from build123d import *

# Parameters (mm, degrees)
SKETCH1_R                 = 8
SKETCH1_R_2               = 11
BOSS_EXTRUDE1_DEPTH       = 5
BOSS_EXTRUDE2_DEPTH       = 11
BOSS_EXTRUDE3_OUTLINE_R   = 1.6
BOSS_EXTRUDE3_OUTLINE_R_2 = 2.1
BOSS_EXTRUDE3_DEPTH       = 3
SKETCH3_W                 = 15
SKETCH3_H                 = 38.75
CUT_EXTRUDE1_DEPTH        = 3
BOSS_EXTRUDE4_REACH       = 120.779
CUT_EXTRUDE3_START        = 3
CUT_EXTRUDE3_OUTLINE_R    = 1.6
CUT_EXTRUDE3_DEPTH        = 5.935416332


# Read off the part's stored shape, not the designer's step: Boss-Extrude3, Cut-Extrude3
with BuildPart() as part:
    # Sketch1 → Boss-Extrude1 (new body)
    with BuildSketch(Plane.XY):
        Polygon((-24, 15), (0, 15), (0, 0), (93, 0), (93, 102.7), (0, 102.7), (0, 30), (-24, 30), align=None)
        with Locations((15, 10.5)):
            Circle(SKETCH1_R, mode=Mode.SUBTRACT)
        with Locations((70, 72)):
            Circle(SKETCH1_R_2, mode=Mode.SUBTRACT)
    extrude(amount=BOSS_EXTRUDE1_DEPTH)

    # Sketch2 → Boss-Extrude2 (add)
    with BuildSketch(Plane(origin=(-11, 0, 0), x_dir=(0, 0, -1), z_dir=(1, 0, 0))):
        Polygon((-6.40446571, 53.75), (-6.40446571, 33.5), (-6.40446571, 30), (0, 30), (0, 53.75), align=None)
    extrude(amount=BOSS_EXTRUDE2_DEPTH)

    # Boss-Extrude3 outline → Boss-Extrude3 (add)
    with BuildSketch(Plane(origin=(-11, 0, 0), x_dir=(0, 0, -1), z_dir=(1, 0, 0))):
        Polygon((-65.7, 15), (-5, 15), (-5, 30), (-6.40446571, 30), (-6.40446571, 53.75), (-65.7, 53.75), align=None)
        with Locations((-25.458037139, 18.009888358)):
            Circle(BOSS_EXTRUDE3_OUTLINE_R, mode=Mode.SUBTRACT)
        with Locations((-33.128928451, 20.361955525)):
            Circle(BOSS_EXTRUDE3_OUTLINE_R_2, mode=Mode.SUBTRACT)
        with BuildLine():
            ThreePointArc((-36.471534651, 41.421088598), (-34.422063775, 42.316430041), (-32.214396715, 42.674443066))
            add(Edge.make_bspline(
                [(-32.214396715, 42.674443066), (-32.258484047, 42.672889926), (-32.30288803, 42.678244048), (-32.383949881, 42.711721435), (-32.420720422, 42.742067925), (-32.450943892, 42.825768035), (-32.442187299, 42.872669516), (-32.401895098, 42.950423281), (-32.37149194, 42.983188581), (-32.336739051, 43.010347732)],
                knots=[0, 0, 0, 0, 0.25, 0.25, 0.5, 0.5, 0.75, 0.75, 1, 1, 1, 1], degree=3))
            ThreePointArc((-32.336739051, 43.010347732), (-12.84214513, 33.068927831), (-32.99665635, 24.544451349))
            add(Edge.make_bspline(
                [(-32.99665635, 24.544451349), (-33.029388791, 24.574028225), (-33.057393425, 24.608892702), (-33.092046693, 24.689435058), (-33.097377316, 24.736767464), (-33.061272852, 24.818024197), (-33.022299349, 24.845743133), (-32.93918463, 24.87327764), (-32.894502735, 24.8754612), (-32.850648228, 24.870765952)],
                knots=[0, 0, 0, 0, 0.25, 0.25, 0.5, 0.5, 0.75, 0.75, 1, 1, 1, 1], degree=3))
            ThreePointArc((-32.850648228, 24.870765952), (-35.02712744, 25.385455582), (-37.007457913, 26.424810377))
            ThreePointArc((-37.007457913, 26.424810377), (-39.660439788, 25.039720747), (-38.589504277, 27.83433758))
            ThreePointArc((-38.589504277, 27.83433758), (-40.824282289, 34.06892783), (-38.150161467, 40.128088348))
            ThreePointArc((-38.150161467, 40.128088348), (-39.018876857, 42.992022649), (-36.471534651, 41.421088598))
        make_face(mode=Mode.SUBTRACT)
        with Locations((-11.766421235, 25.275537259)):
            Circle(BOSS_EXTRUDE3_OUTLINE_R, mode=Mode.SUBTRACT)
        with Locations((-9.414354068, 32.946428571)):
            Circle(BOSS_EXTRUDE3_OUTLINE_R_2, mode=Mode.SUBTRACT)
        with Locations((-11.212849807, 40.765648901)):
            Circle(BOSS_EXTRUDE3_OUTLINE_R, mode=Mode.SUBTRACT)
        with Locations((-32.170114611, 47.191615903)):
            Circle(BOSS_EXTRUDE3_OUTLINE_R_2, mode=Mode.SUBTRACT)
        with Locations((-24.350894282, 48.990111642)):
            Circle(BOSS_EXTRUDE3_OUTLINE_R, mode=Mode.SUBTRACT)
    extrude(amount=BOSS_EXTRUDE3_DEPTH)

    # Sketch3 → Cut-Extrude1 (cut)
    with BuildSketch(Plane(origin=(-8, 0, 0), x_dir=(0, 0, -1), z_dir=(1, 0, 0))):
        with Locations((-58.2, 34.375)):
            Rectangle(SKETCH3_W, SKETCH3_H)
    extrude(amount=-CUT_EXTRUDE1_DEPTH, mode=Mode.SUBTRACT)

    # Boss-Extrude4: up to this face of the body (flat: up to its plane)
    boss_extrude4_end = Plane(part.part.faces().sort_by_distance((-10.666861144, 15, 16.018028005))[0])
    # Sketch4 → Boss-Extrude4 (add, up to the picked face)
    with BuildSketch(Plane(origin=(0, 53.75, 0), x_dir=(1, 0, 0), z_dir=(0, 1, 0)), mode=Mode.PRIVATE) as boss_extrude4_sk1:
        with BuildLine():
            Line((8.727174225, -5), (-8, -5))
            Line((-8, -5), (-8, -17.898489496))
            ThreePointArc((-8, -17.898489496), (-1.439507221, -9.110934277), (8.727174225, -5))
        make_face()
    boss_extrude4_tool1 = split(extrude(boss_extrude4_sk1.sketch, amount=-BOSS_EXTRUDE4_REACH, mode=Mode.PRIVATE), bisect_by=boss_extrude4_end, keep=Keep.BOTH, mode=Mode.PRIVATE)
    add(boss_extrude4_tool1.solids().sort_by(Axis((-3.750344, 53.75, 8.522384), (0, -1, 0)))[0])

    # Cut-Extrude3 outline → Cut-Extrude3 (cut)
    with BuildSketch(Plane(origin=(-11, 0, 0), x_dir=(0, 0, -1), z_dir=(1, 0, 0)).offset(CUT_EXTRUDE3_START)):
        with BuildLine():
            ThreePointArc((-19, 22.972764576), (-12.834444956, 33.5), (-19, 44.027235424))
            Line((-19, 44.027235424), (-19, 22.972764576))
        make_face()
        with Locations((-11.766421235, 25.275537259)):
            Circle(CUT_EXTRUDE3_OUTLINE_R)
        with Locations((-11.212849807, 40.765648901)):
            Circle(CUT_EXTRUDE3_OUTLINE_R)
    extrude(amount=CUT_EXTRUDE3_DEPTH, mode=Mode.SUBTRACT)


solid = part.part
Design review of the part built by this model. Coordinates are the model's own, in mm. A direction names the side the tool comes from. Coordinates: 2 decimals unless noted, no trailing zeros. Order: outer loops, then holes, each group sorted by start corner. A loop starts at its lowest first (then second) coordinate and runs counter-clockwise, first axis right, second up. Notation, with made-up numbers: (75.25, -29.5) -> (119.25, -29.5) arc R21 cw to (119.25, 9.5) -> close; hole circle Ø5 at (4, 41.25). An arc over 180 degrees is marked (long way). One line per item, written item: value.
1) We need section A-A, the plane y = 10.5. Give the boundary of the cut face in (x, z), then the cut area to 3 significant figures.
Output values:
outline: (0, 0) -> (7, 0) -> (7, 5) -> (0, 5) -> close; (23, 0) -> (93, 0) -> (93, 5) -> (23, 5) -> close
area: 385 mm2
2) Machinability: for faces 4 (the face through (-8, 33, 9)), 5 (the face through (-9.521, 33.974, 40.827)), 6 (the face through (-8, 35, 42)), which of the approach directions +Z, -Z, +X, -X, +Y, -Y give a long, thin tool a straight path to every point of the face, cutting with its end or side? Answer none if there is none.
Output values:
face 4: -X
face 5: +X, -X
face 6: +Z, +X, +Y, -Y
3) We need section D-D, the plane z = 47. Give the boundary of the cut face in (x, y), then the cut area to 3 significant figures.
Output values:
outline: (-11, 15) -> (-8, 15) -> (-8, 53.75) -> (-11, 53.75) -> close
area: 116 mm2
4) Clearance check with flat-ended pins moving along their axes: P1, Ø3, axis at x = 58.5, y = 40, coming from the +Z side; P2, Ø3.5, axis at y = 48.99, z = 24.35, coming from the -X side; P3, Ø18.5, axis at x = 15, y = 10.5, coming from the +Z side; P4, Ø11.5, axis at y = 29, z = 24.5, coming from the -X side. State where each tip first meets the part, or that it passes through.
Output values:
P1: stops at z = 5
P2: stops at x = -11
P3: stops at z = 5.29
P4: passes through
5) We need section B-B, the plane x = 15. Give the boundary of the cut face in (y, z), then the cut area to 4 significant figures.
Output values:
outline: (0, 0) -> (2.5, 0) -> (2.5, 5) -> (0, 5) -> close; (18.5, 0) -> (102.7, 0) -> (102.7, 5) -> (18.5, 5) -> close
area: 433.5 mm2
6) Draft analysis for pull direction X (two halves, no side actions). For faces 1 (the face through (0, 79, 2)), 2 (the face through (13.27, 2.69, 2.46)), 3 (the face through (-7.588, 40.153, 9.735)), state which applies: +X half, -X half, draft (parallel to the pull), parting line (faces both ways), or undercut.
Output values:
face 1: -X half
face 2: undercut
face 3: draft
7) To check wall thickness, follow probe 1 along Z at (x, y) = (-9.9, 33.5); probe 2 along X at (y, z) = (52, 44); probe 3 along Z at (x, y) = (71, 41). State the ranges of each line that lie inside material, in increasing order. Write a range as [from, to].
Output values:
probe 1: z = [0, 7.39], [11.44, 12.83], [40.83, 50.7]
probe 2: x = [-11, -8]
probe 3: z = [0, 5]
8) We need section C-C, the plane z = 15. Give the boundary of the cut face in (x, y), then the cut area to 3 significant figures.
Output values:
outline: (-11, 15) -> (-6.61, 15) -> (-6.61, 26.6) -> (-11, 26.6) -> close; (-11, 40.4) -> (-6.61, 40.4) -> (-6.61, 53.75) -> (-11, 53.75) -> close
area: 110 mm2
